```python
from build123d import *

# Parameters (mm, degrees)
F1_DEPTH = 1.6


# Not quite as in the source:
# - a feature names something its author has since deleted; it is built from what else it names


with BuildPart() as f1:
    # F0 (on Top) → F1 (new body, symmetric)
    with BuildSketch(Plane.XY):
        with BuildLine():
            Line((-21, 3.2), (-21, 0))
            ThreePointArc((-21, 0), (-20.1245739235, -6.0001270317), (-17.5712833908, -11.5))
            Line((-17.5712833908, -11.5), (0, -11.5))
            Line((0, -11.5), (17.5712833908, -11.5))
            ThreePointArc((17.5712833908, -11.5), (20.1245739235, -6.0001270317), (21, 0))
            Line((21, 0), (19, 0))
            Line((19, 0), (19, 3.2))
            Line((19, 3.2), (11, 3.2))
            Line((11, 3.2), (11, 0))
            Line((11, 0), (3, 0))
            Line((3, 0), (3, 3.2))
            Line((3, 3.2), (-5, 3.2))
            Line((-5, 3.2), (-5, 0))
            Line((-5, 0), (-13, 0))
            Line((-13, 0), (-13, 3.2))
            Line((-13, 3.2), (-21, 3.2))
        make_face()
    extrude(amount=F1_DEPTH, both=True)


solid = f1.part
```
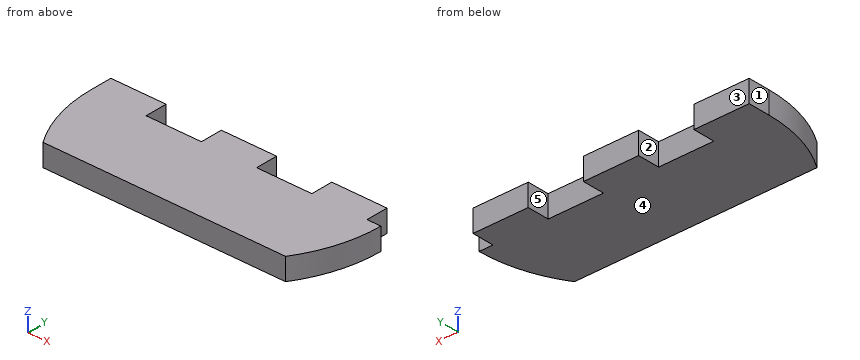
The model under review builds one solid part; all positions refer to its coordinate system, in mm. Face numbers are marked on the shaded views. A direction names the side the tool comes from. Round coordinates to 2 decimals unless told otherwise and drop trailing zeros. Loops run counter-clockwise (first coordinate to the right, second up) from the corner with the lowest first, then second, coordinate; pieces in that order, holes last. Notation, with made-up numbers: (-14.5, 23.25) - (-0.5, 23.25) arc R22 cw to (-0.5, 47.25) - close; hole circle Ø4 at (-35, 88). An arc over 180 degrees is marked (long way). Write each question's results on one line, items separated by ' | '. Start each with the question number.
Q1. Wall thickness on line 1 along X through (y, z) = (0.75, 0.35); line 2 along Y through (x, z) = (5.5, -1.3); line 3 along X through (y, z) = (-1.5, -0.1): over which ranges is each line inside the solid? List them lowest first. Write a range as [from, to].
Q2. Take a section at A-A on y = 2. Give the boundary of the cut face in (x, z), plus the area to 3 significant figures.
Q3. Take a section at D-D on y = -9.25. Give the boundary of the cut face in (x, z), plus the area to 3 significant figures.
Q4. Insertion check: P1, Ø1, axis at y = 1, z = 0.5, coming from the +X side; P2, Ø1.5, axis at y = -2, z = 0, coming from the -X side; P3, Ø1, axis at x = 20, z = 1, coming from the +Y side. Each pin has a flat end and moves straight along its axis. Give the tip position at first contact, or say it passes through.
Q5. Take a section at C-C on x = -10. Give the boundary of the cut face in (y, z).
Q6. Draft analysis for pull direction X (two halves, no side actions). For the marked faces 1, 2 and 3, state which applies: pulls with the +X half, pulls with the -X half, needs draft (parallel to the pull), parting line crosses it, or undercut.
Q7. Tool access review of the marked faces 4 and 5: name each direction out of +Z, -Z, +X, -X, +Y, -Y from which nothing blocks a thin tool from reaching the whole face with its end or side.
Q8. Take a section at B-B on z = 0.25. Give the boundary of the cut face in (x, y), plus the area to 3 significant figures.
Data:
1) line 1: x = [-21, -13], [-5, 3], [11, 19] | line 2: y = [-11.5, 0] | line 3: x = [-20.95, 20.95]
2) outline: (-21, -1.6) - (-13, -1.6) - (-13, 1.6) - (-21, 1.6) - close; (-5, -1.6) - (3, -1.6) - (3, 1.6) - (-5, 1.6) - close; (11, -1.6) - (19, -1.6) - (19, 1.6) - (11, 1.6) - close | area: 76.8 mm²
3) outline: (-18.85, -1.6) - (18.85, -1.6) - (18.85, 1.6) - (-18.85, 1.6) - close | area: 121 mm²
4) P1: stops at x = 19 | P2: stops at x = -20.96 | P3: stops at y = 0
5) outline: (-11.5, -1.6) - (0, -1.6) - (0, 1.6) - (-11.5, 1.6) - close
6) face 1: pulls with the -X half | face 2: undercut | face 3: needs draft
7) face 4: -Z, +X, -X, +Y, -Y | face 5: +Z, -Z, +Y
8) outline: (-21, 0) arc R21 ccw to (-17.57, -11.5) - (17.57, -11.5) arc R21 ccw to (21, 0) - (19, 0) - (19, 3.2) - (11, 3.2) - (11, 0) - (3, 0) - (3, 3.2) - (-5, 3.2) - (-5, 0) - (-13, 0) - (-13, 3.2) - (-21, 3.2) - close | area: 534 mm²
